Could you check a few things on this model? Use its own coordinates, in mm. Round coordinates to 2 decimals unless told otherwise and drop trailing zeros. Write each loop counter-clockwise with the first axis right and the second up, starting at its lowest first coordinate (ties: lowest second). Pieces come first, ordered by that corner, then holes. Notation, with made-up numbers: (-5, 6.5) - (29, 6.5) arc R31 ccw to (29, 45.5) - close; hole circle Ø10 at (-31.5, -18.75). An arc over 180 degrees is marked (long way). Put each result on its own line as item: value.
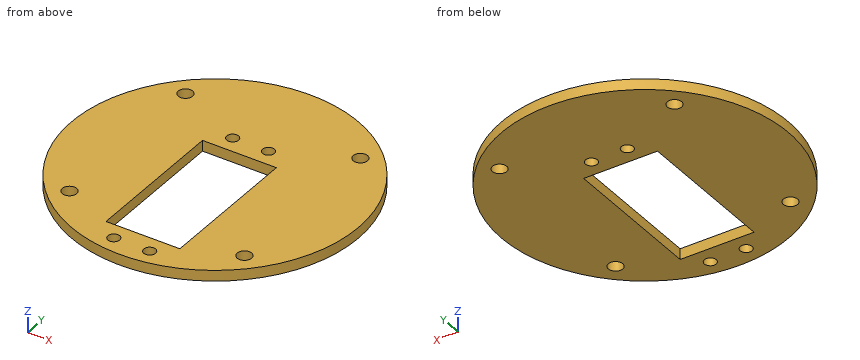
from build123d import *

# Parameters (mm, degrees)
PLATE_D80_HOLES_D4_DIAGONAL69_R      = 40
PLATE_D80_HOLES_D4_DIAGONAL69_R_2    = 2
PLATE_3MM_DEPTH                      = 3
SERVO_HOUSING_THROUGH_CUT_START      = -0.1
SERVO_HOUSING_PROFILE_40P6X20P6_W    = 20.6
SERVO_HOUSING_PROFILE_40P6X20P6_H    = 40.6
SERVO_HOUSING_THROUGH_CUT_DEPTH      = 3.2
SERVO_4XD3P3_THROUGH_HOLES_START     = -0.1
SERVO_EARS_50X10_CENTERED_ON_SHAFT_R = 1.65
SERVO_4XD3P3_THROUGH_HOLES_DEPTH     = 3.2


with BuildPart() as part:
    # Plate_D80_Holes_D4_Diagonal69 → Plate_3mm (new body)
    with BuildSketch(Plane.XY):
        Circle(PLATE_D80_HOLES_D4_DIAGONAL69_R)
        with Locations((-24.395183951, -24.395183951)):
            Circle(PLATE_D80_HOLES_D4_DIAGONAL69_R_2, mode=Mode.SUBTRACT)
        with Locations((-24.395183951, 24.395183951)):
            Circle(PLATE_D80_HOLES_D4_DIAGONAL69_R_2, mode=Mode.SUBTRACT)
        with Locations((24.395183951, -24.395183951)):
            Circle(PLATE_D80_HOLES_D4_DIAGONAL69_R_2, mode=Mode.SUBTRACT)
        with Locations((24.395183951, 24.395183951)):
            Circle(PLATE_D80_HOLES_D4_DIAGONAL69_R_2, mode=Mode.SUBTRACT)
    extrude(amount=PLATE_3MM_DEPTH)

    # Servo_Housing_Profile_40p6x20p6 → Servo_Housing_Through_Cut (cut)
    with BuildSketch(Plane.XY.offset(SERVO_HOUSING_THROUGH_CUT_START)):
        with Locations((0, -10)):
            Rectangle(SERVO_HOUSING_PROFILE_40P6X20P6_W, SERVO_HOUSING_PROFILE_40P6X20P6_H)
    extrude(amount=SERVO_HOUSING_THROUGH_CUT_DEPTH, mode=Mode.SUBTRACT)

    # Servo_Ears_50x10_Centered_on_Shaft → Servo_4xD3p3_Through_Holes (cut)
    with BuildSketch(Plane.XY.offset(SERVO_4XD3P3_THROUGH_HOLES_START)):
        with Locations((-5, -35)):
            Circle(SERVO_EARS_50X10_CENTERED_ON_SHAFT_R)
        with Locations((-5, 15)):
            Circle(SERVO_EARS_50X10_CENTERED_ON_SHAFT_R)
        with Locations((5, -35)):
            Circle(SERVO_EARS_50X10_CENTERED_ON_SHAFT_R)
        with Locations((5, 15)):
            Circle(SERVO_EARS_50X10_CENTERED_ON_SHAFT_R)
    extrude(amount=SERVO_4XD3P3_THROUGH_HOLES_DEPTH, mode=Mode.SUBTRACT)


solid = part.part
(1) Imagine slicing it at C-C, the plane z = 2.45. Give the number of separate pieces and of enclosed holes in the cut face, then the cut area to 3 significant figures.
Values found:
separate pieces: 1
enclosed holes: 9
area: 4,110 mm^2
(2) Imagine slicing it at A-A, the plane y = 0. List the corners of the cut face in (x, z) for me, then the cut area to 3 significant figures.
Values found:
outline: (-40, 0) - (-10.3, 0) - (-10.3, 3) - (-40, 3) - close; (10.3, 0) - (40, 0) - (40, 3) - (10.3, 3) - close
area: 178 mm^2
(3) Imagine slicing it at B-B, the plane x = 0. List the corners of the cut face in (y, z) for me, then the cut area to 3 significant figures.
Values found:
outline: (-40, 0) - (-30.3, 0) - (-30.3, 3) - (-40, 3) - close; (10.3, 0) - (40, 0) - (40, 3) - (10.3, 3) - close
area: 118 mm^2
(4) I'm going to push flat-ended pins straight in: pin 1 (0.9 mm diameter, centred on y = -18.5, z = 2, fed in from +X); pin 2 (12 mm diameter, centred on x = -20, y = 21.5, fed in from -Z); pin 3 (2.5 mm diameter, centred on x = -24.4, y = -24.4, fed in from -Z); pin 4 (0.9 mm diameter, centred on x = -3, z = 1, fed in from -Y). Where does each tip first touch, or does it pass through?
Values found:
pin 1: stops at x = 35.7
pin 2: stops at z = 0
pin 3: passes through
pin 4: stops at y = -39.92
(5) Please list where these lines run through material, in increasing order: probe 1 along Y at (x, z) = (0.5, 2.55); probe 2 along X at (y, z) = (15, 0.55); probe 3 along X at (y, z) = (-35, 1.75). Write a range as from..to.
Values found:
probe 1: y = -40..-30.3, 10.3..40
probe 2: x = -37.08..-6.65, -3.35..3.35, 6.65..37.08
probe 3: x = -19.36..-6.65, -3.35..3.35, 6.65..19.36
(6) Imagine slicing it at D-D, the plane y = -35. List the corners of the cut face in (x, z) for me.
Values found:
outline: (-19.36, 0) - (-6.65, 0) - (-6.65, 3) - (-19.36, 3) - close; (-3.35, 0) - (3.35, 0) - (3.35, 3) - (-3.35, 3) - close; (6.65, 0) - (19.36, 0) - (19.36, 3) - (6.65, 3) - close
